Study the drawing (mm; zero at the part's minimum x, y, z) and answer. A direction names the side the tool comes from. Give positions to 0.01 mm unless a question says otherwise; leave off trailing zeros. Order: outer loops, then holes, each group sorted by start corner. A loop starts at its lowest first (then second) coordinate and runs counter-clockwise, first axis right, second up. Notation, with made-up numbers: (27.25, 56.5) - (66.25, 56.5) arc R23 cw to (66.25, 64.5) - close; hole circle Ø4 at (83, -15). An arc over 180 degrees is marked (long way). Return JSON: item names as keys, results as strings.
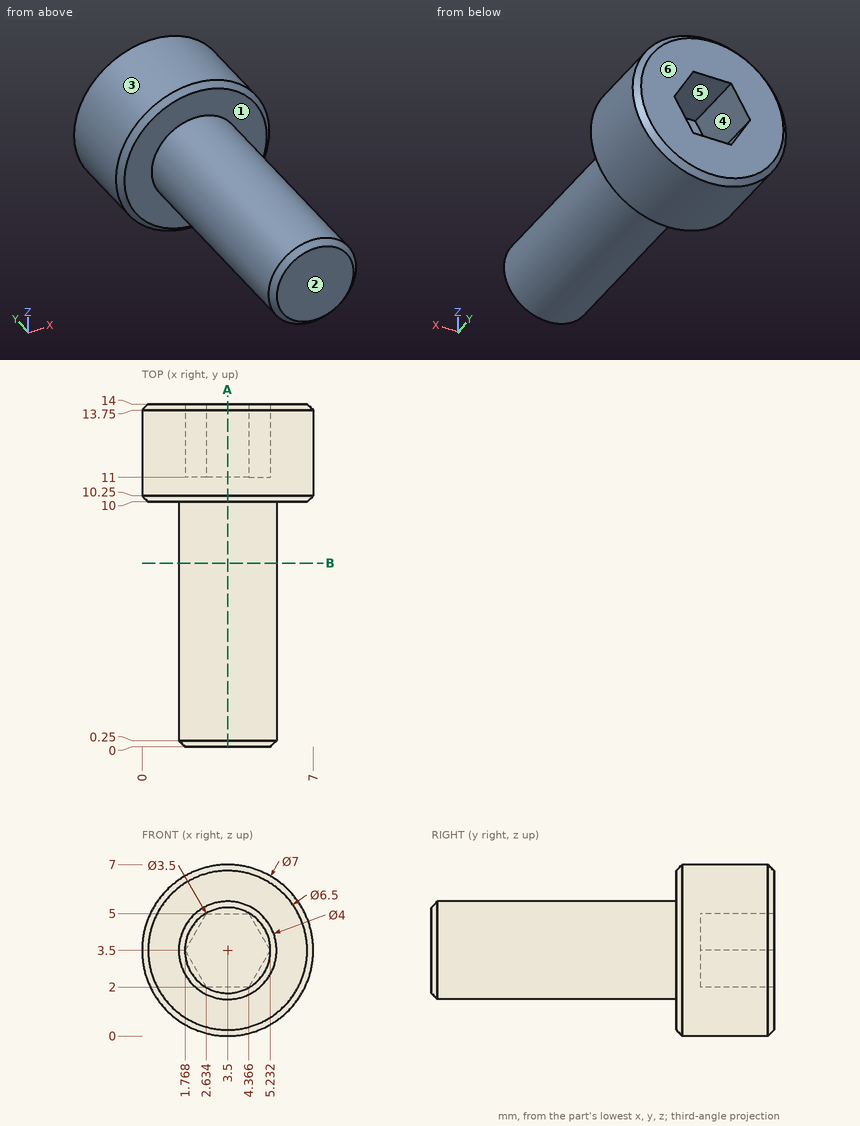
Q1. Determine the mould class of the marked faces 3, 4, 5 and 6 for opening direction X: released by +X, released by -X, zero draft, split by the parting line, or undercut.
Values:
{"face 3": "split by the parting line", "face 4": "undercut", "face 5": "undercut", "face 6": "zero draft"}
Q2. For the marked faces 1 and 2, determine the directions among +Z, -Z, +X, -X, +Y, -Y from which every point of the face is accessible in a straight line to the end or side of a thin tool.
Values:
{"face 1": "-Y", "face 2": "+Z, -Z, +X, -X, -Y"}
Q3. Given pin 1 (2 mm diameter, centred on x = 3.5, z = 2, fed in from -Y); pin 2 (2 mm diameter, centred on x = 2, y = 8, fed in from -Z); pin 3 (1.5 mm diameter, centred on x = 5.5, z = 1.5, fed in from -Y); pin 4 (0.9 mm diameter, centred on x = 4, z = 3.5, fed in from +Y), each flat-ended and moving along its own axis, determine where each tip first touches the part or whether it passes through.
Values:
{"pin 1": "stops at y = 0", "pin 2": "stops at z = 1.56", "pin 3": "stops at y = 10", "pin 4": "stops at y = 11"}
Q4. Consider L1, parallel to Y at x = 6, z = 3.25; L2, parallel to Z at x = 3.5, y = 7.5; L3, parallel to X at y = 12, z = 2.75. Determine where each line is inside the solid, lowest interval first.
Values:
{"L1": "y = 10 to 14", "L2": "z = 1.5 to 5.5", "L3": "x = 0.08 to 2.2, 4.8 to 6.92"}
Q5. A cutting plane is placed at A-A (x = 3.5). Write down the section's boundary in (y, z), and give its area (3 significant figures).
Values:
{"outline": "(0, 1.75) - (0.25, 1.5) - (10, 1.5) - (10, 0.25) - (10.25, 0) - (13.75, 0) - (14, 0.25) - (14, 2) - (11, 2) - (11, 5) - (14, 5) - (14, 6.75) - (13.75, 7) - (10.25, 7) - (10, 6.75) - (10, 5.5) - (0.25, 5.5) - (0, 5.25) - close", "area": "58.8 mm²"}
Q6. A cutting plane is placed at B-B (y = 7.5). Write down the section's boundary in (x, z).
Values:
{"outline": "circle Ø4 at (3.5, 3.5)"}
